For this review, use the dimensioned drawing (mm, ordinates from the lowest corner) and the shaded views. A direction names the side the tool comes from. Round coordinates to 2 decimals unless told otherwise and drop trailing zeros. Write each loop counter-clockwise with the first axis right and the second up, starting at its lowest first coordinate (ties: lowest second). Pieces come first, ordered by that corner, then holes. Notation, with made-up numbers: (-20, 21.5) - (-2, 21.5) arc R24 cw to (-2, 38.5) - close; hole circle Ø2 at (36.5, 67). An arc over 180 degrees is marked (long way). Return JSON: item names as keys, results as strings.
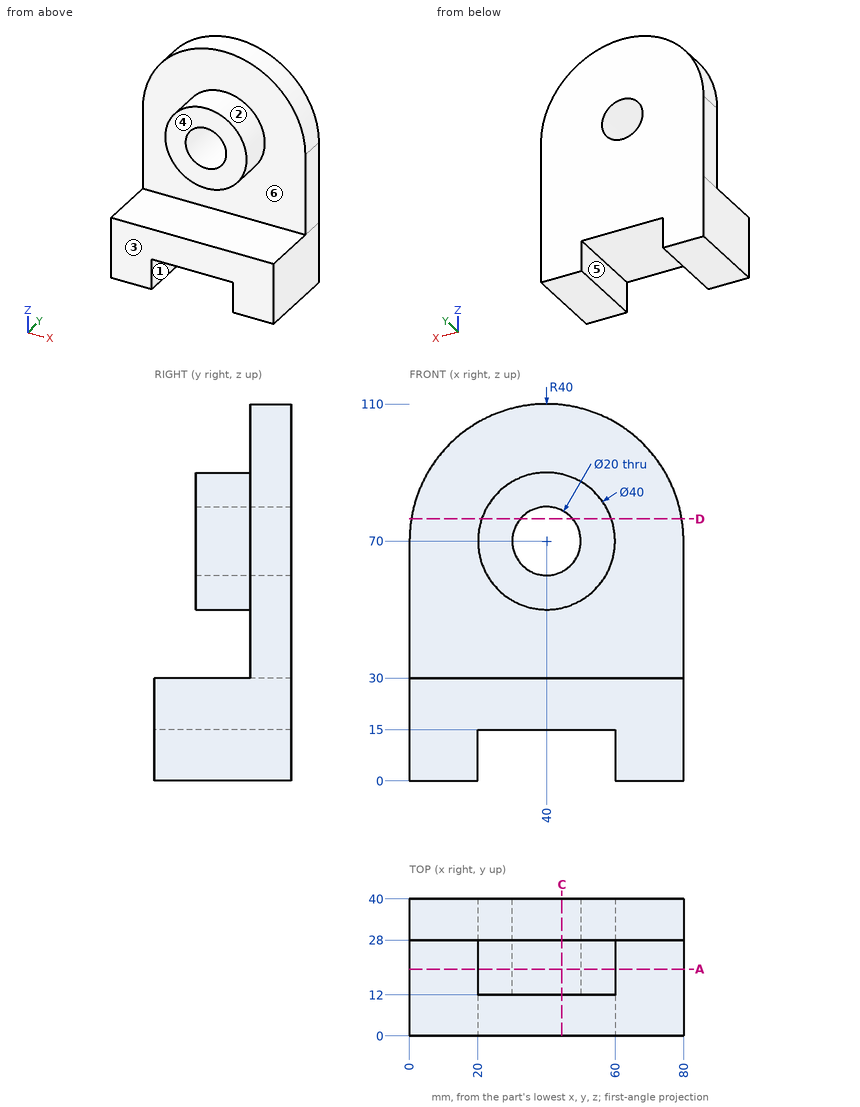
(1) Add section C-C (x = 44.5). Write out the cut boundary in (y, z), plus the area to 3 significant figures.
Filled in:
{"outline": "(0, 15) - (40, 15) - (40, 61.07) - (12, 61.07) - (12, 50.51) - (28, 50.51) - (28, 30) - (0, 30) - close; (12, 78.93) - (40, 78.93) - (40, 109.75) - (28, 109.75) - (28, 89.49) - (12, 89.49) - close", "area": "1,680 mm2"}
(2) Clearance check with flat-ended pins moving along their axes: pin 1 Ø12 at (x, y) = (20, 35) entering from +Z; pin 2 Ø3 at (x, y) = (10.5, 30.5) entering from +Z; pin 3 Ø12 at (x, z) = (40, 70) entering from +Y; pin 4 Ø5 at (x, y) = (12.5, 20.5) entering from +Z. State where each tip first meets the part, or that it passes through.
Filled in:
{"pin 1": "stops at z = 107.47", "pin 2": "stops at z = 98.57", "pin 3": "passes through", "pin 4": "stops at z = 30"}
(3) Mouldability with a two-part tool opening along X and no side actions: class the marked faces 1, 2 and 3 as released by +X, released by -X, zero draft, split by the parting line, or undercut.
Filled in:
{"face 1": "undercut", "face 2": "split by the parting line", "face 3": "zero draft"}
(4) For the marked faces 4, 5 and 6, list the 3-axis set-ups (+Z, -Z, +X, -X, +Y, -Y) from which the entire face can be reached by the end or side of a thin tool; tool diameter is ignored.
Filled in:
{"face 4": "+Z, +X, -X, -Y", "face 5": "-Z, +Y, -Y", "face 6": "-Y"}
(5) Add section A-A (y = 19.5). Write out the cut boundary in (x, z), plus the area to 3 significant figures.
Filled in:
{"outline": "(0, 0) - (20, 0) - (20, 15) - (60, 15) - (60, 0) - (80, 0) - (80, 30) - (0, 30) - close; circle Ø40 at (40, 70); hole circle Ø20 at (40, 70)", "area": "2,740 mm2"}
(6) Wall thickness on line 1 (Z direction, x = 48, y = 18); line 2 (X direction, y = 14, z = 8.5); line 3 (Y direction, x = 45, z = 43): over which ranges is each line inside the solid? List them lowest first.
Filled in:
{"line 1": "z = 15 to 30, 51.67 to 64, 76 to 88.33", "line 2": "x = 0 to 20, 60 to 80", "line 3": "y = 28 to 40"}
(7) Add section D-D (z = 76.5). Write out the cut boundary in (x, y).
Filled in:
{"outline": "(0.53, 28) - (21.09, 28) - (21.09, 12) - (32.4, 12) - (32.4, 40) - (0.53, 40) - close; (47.6, 12) - (58.91, 12) - (58.91, 28) - (79.47, 28) - (79.47, 40) - (47.6, 40) - close"}
